Verification items for the finished model (mm, model axes). Face numbers are marked on the shaded views. A direction names the side the tool comes from. Round coordinates to 2 decimals unless told otherwise and drop trailing zeros. Order: outer loops, then holes, each group sorted by start corner. A loop starts at its lowest first (then second) coordinate and runs counter-clockwise, first axis right, second up. Notation, with made-up numbers: M 6,-17 L 33,-17 A23 cw 33,17 Z; hole C 66.5,22 d3. An arc over 180 degrees is marked long. One line per item, written item: value. Start each with the question number.
from build123d import *

# Parameters (mm, degrees)
SKETCH_W        = 50
SKETCH_H        = 35
PAD_DEPTH       = 3
SKETCH002_W     = 45
SKETCH002_H     = 30
PAD001_DEPTH    = 1.5
SKETCH003_W     = 43
SKETCH003_H     = 28
POCKET001_DEPTH = 2.5
FILLET_R        = 2.9
FILLET001_R     = 1
SKETCH005_R     = 2.5
PAD002_DEPTH    = 5
SKETCH004_R     = 2.5
PAD003_DEPTH    = 5
SKETCH006_R     = 1.75
POCKET_DEPTH    = 5
SKETCH007_R     = 1.75
POCKET002_DEPTH = 5
CHAMFER_SIZE    = 1.5
CHAMFER001_SIZE = 1.5


with BuildPart() as part:
    # Sketch → Pad (new body)
    with BuildSketch(Plane.XY):
        Rectangle(SKETCH_W, SKETCH_H)
    extrude(amount=PAD_DEPTH)

    # Sketch002 → Pad001 (join)
    with BuildSketch(Plane.XY.offset(3)):
        Rectangle(SKETCH002_W, SKETCH002_H)
    extrude(amount=PAD001_DEPTH)

    # Sketch003 (on Face11 of Pad001) → Pocket001 (cut)
    with BuildSketch(Plane.XY.offset(4.5)):
        Rectangle(SKETCH003_W, SKETCH003_H)
    extrude(amount=-POCKET001_DEPTH, mode=Mode.SUBTRACT)

    # Fillet
    fillet_edges = [part.edges().sort_by_distance(p)[0] for p in [
        (0, 17.5, 0),
        (-25, 17.5, 1.5),
        (-25, 0, 0),
        (-25, -17.5, 1.5),
        (0, -17.5, 0),
        (25, -17.5, 1.5),
        (25, 0, 0),
        (25, 17.5, 1.5),
    ]]
    fillet(fillet_edges, radius=FILLET_R)

    # Fillet001
    fillet001_edges = [part.edges().sort_by_distance(p)[0] for p in [
        (-21.5, -14, 3.25),
        (22.5, -15, 3.75),
        (22.5, 15, 3.75),
        (-22.5, 15, 3.75),
        (-22.5, -15, 3.75),
        (21.5, 14, 3.25),
        (-21.5, 14, 3.25),
        (21.5, -14, 3.25),
    ]]
    fillet(fillet001_edges, radius=FILLET001_R)

    # Sketch005 → Pad002 (join)
    with BuildSketch(Plane.XY):
        with Locations((-19.25, 11.75)):
            Circle(SKETCH005_R)
    extrude(amount=PAD002_DEPTH)

    # Sketch004 (on Face35 of Fillet001) → Pad003 (join)
    with BuildSketch(Plane(origin=(0, 0, 0), x_dir=(1, 0, 0), z_dir=(0, 0, -1))):
        with Locations((19.25, 11.75)):
            Circle(SKETCH004_R)
    extrude(amount=-PAD003_DEPTH)

    # Sketch006 (on Face48 of Pad003) → Pocket (cut)
    with BuildSketch(Plane(origin=(0, 0, 0), x_dir=(1, 0, 0), z_dir=(0, 0, -1))):
        with Locations((-19.25, -11.75)):
            Circle(SKETCH006_R)
    extrude(amount=-POCKET_DEPTH, mode=Mode.SUBTRACT)

    # Sketch007 (on Face48 of Pocket) → Pocket002 (cut)
    with BuildSketch(Plane(origin=(0, 0, 0), x_dir=(1, 0, 0), z_dir=(0, 0, -1))):
        with Locations((19.25, 11.75)):
            Circle(SKETCH007_R)
    extrude(amount=-POCKET002_DEPTH, mode=Mode.SUBTRACT)

    # Chamfer
    chamfer_edges = [part.edges().sort_by_distance(p)[0] for p in [
        (-21, 11.75, 0),
    ]]
    chamfer(chamfer_edges, length=CHAMFER_SIZE)

    # Chamfer001
    chamfer001_edges = [part.edges().sort_by_distance(p)[0] for p in [
        (17.5, -11.75, 0),
    ]]
    chamfer(chamfer001_edges, length=CHAMFER001_SIZE)


solid = part.part
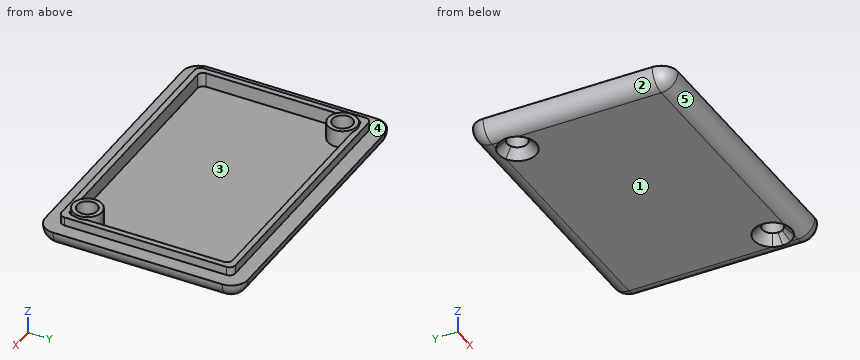
1. Draft check along X on the marked faces 1, 2 and 3. Enter one of: released by +X, released by -X, zero draft, split by the parting line, or undercut.
2. Tool access check on the marked faces 4 and 5. Record the directions out of +Z, -Z, +X, -X, +Y, -Y that give a thin tool (end or side, any length) a straight path to the whole face; none if there is none.
3. Section check A-A (z = 3.55). Record the cut outline in (x, y), and give its area (3 significant figures).
4. Scan lines: line 1 along Y through (x, z) = (19.25, 2.9); line 2 along Y through (x, z) = (-19.25, 3.4); line 3 along X through (y, z) = (-11.75, 3.3). Record each from-to range of solid material in increasing order.
5. Section check C-C (y = -3.5). Record the cut outline in (x, z), and give its area (3 significant figures).
6. Depth check by flat-ended pin: pin 1 (10.5 mm diameter, centred on x = -8.5, y = -3.5, fed in from +Z); pin 2 (3 mm diameter, centred on x = -19.25, y = 11.75, fed in from +Z); pin 3 (0.8 mm diameter, centred on y = -4.5, z = 4, fed in from -X); pin 4 (1.2 mm diameter, centred on y = -6, z = 4, fed in from +X). Enter the tip coordinate at first touch or a pass-through.
7. Section check B-B (x = 15.5). Record the cut outline in (y, z).
Geometry check:
1. face 1: zero draft
1. face 2: released by -X
1. face 3: undercut
2. face 4: +Z
2. face 5: -Z, +X, -X, -Y
3. outline: M -22.5,-14 A1 ccw -21.5,-15 L 21.5,-15 A1 ccw 22.5,-14 L 22.5,14 A1 ccw 21.5,15 L -21.5,15 A1 ccw -22.5,14 Z; hole M -21.5,-13 A1 ccw -20.5,-14 L 18.16,-14 A2.5 cw long 21.5,-10.66 L 21.5,13 A1 ccw 20.5,14 L -18.16,14 A2.5 cw long -21.5,10.66 Z; hole M -21.5,12.84 A2.5 cw -20.34,14 L -20.5,14 A1 ccw -21.5,13 Z; hole C -19.25,11.75 d3.5; hole C 19.25,-11.75 d3.5; hole M 20.34,-14 L 20.5,-14 A1 ccw 21.5,-13 L 21.5,-12.84 A2.5 cw Z
3. area: 165 mm²
4. line 1: y = -17.5 to -13.5, -10 to -9.25, 14 to 17.5
4. line 2: y = -15 to -14, 9.25 to 10, 13.5 to 15
4. line 3: x = -22.5 to -21.5, 16.75 to 17.5, 21 to 22.5
5. outline: M -25,2.9 A2.9 ccw -22.1,0 L 22.1,0 A2.9 ccw 25,2.9 L 25,3 L 22.5,3 L 22.5,4.5 L 21.5,4.5 L 21.5,2 L -21.5,2 L -21.5,4.5 L -22.5,4.5 L -22.5,3 L -25,3 Z
5. area: 106 mm²
6. pin 1: stops at z = 2
6. pin 2: passes through
6. pin 3: stops at x = -22.5
6. pin 4: stops at x = 22.5
7. outline: M -17.5,2.9 A2.9 ccw -14.6,0 L 14.6,0 A2.9 ccw 17.5,2.9 L 17.5,3 L 15,3 L 15,4.5 L 14,4.5 L 14,2 L -14,2 L -14,4.5 L -15,4.5 L -15,3 L -17.5,3 Z
